from build123d import *


with BuildPart() as f1:
    # F0 (on Front) → F1 (revolve)
    with BuildSketch(Plane.XZ):
        with BuildLine():
            ThreePointArc((-1.815014, 4.25), (-1.448898, 3.366117), (-0.565014, 3))
            Line((-0.565014, 3), (6.184986, 3))
            Line((6.184986, 3), (6.184986, 3.909007))
            Line((6.184986, 3.909007), (5.934986, 4))
            Line((5.934986, 4), (-0.565014, 4))
            ThreePointArc((-0.565014, 4), (-0.741791, 4.073223), (-0.815014, 4.25))
            Line((-0.815014, 4.25), (-0.815014, 6))
            Line((-0.815014, 6), (-1.815014, 6))
            Line((-1.815014, 6), (-1.815014, 4.25))
        make_face()
    revolve(axis=Axis((-0.667828, 0, 0), (1, 0, 0)))


solid = f1.part
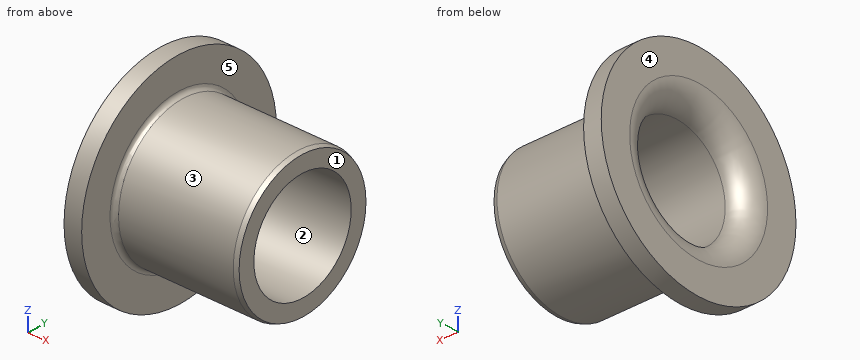
CAD build for the part. Positions are in the model's coordinates, mm. Face numbers are marked on the shaded views. A direction names the side the tool comes from. Give positions to 0.01 mm unless a question says otherwise; leave off trailing zeros. Order: outer loops, then holes, each group sorted by start corner. A loop starts at its lowest first (then second) coordinate and runs counter-clockwise, first axis right, second up. Notation, with made-up numbers: (-31.75, -0.75) - (2.25, -0.75) arc R28 ccw to (2.25, 19.25) - close; hole circle Ø4 at (82, 36.25). An arc over 180 degrees is marked (long way). Answer in a Markdown table with one row per item.
1. Saw through at A-A, the plane y = 0. Give the cut face in (x, z).
Data:
| item | result |
|---|---|
| outline | (-1.82, -6) - (-0.82, -6) - (-0.82, -4.25) arc R0.25 cw to (-0.57, -4) - (5.93, -4) - (6.18, -3.91) - (6.18, -3) - (-0.57, -3) arc R1.25 ccw to (-1.82, -4.25) - close; (-1.82, 4.25) arc R1.25 ccw to (-0.57, 3) - (6.18, 3) - (6.18, 3.91) - (5.93, 4) - (-0.57, 4) arc R0.25 cw to (-0.82, 4.25) - (-0.82, 6) - (-1.82, 6) - close |
2. Saw through at C-C, the plane x = 0.5. Give the cut face in (y, z), plus the area to 3 significant figures.
Data:
| item | result |
|---|---|
| outline | circle Ø8 at (0, 0); hole circle Ø6 at (0, 0) |
| area | 22.0 mm² |
3. Tool access for the marked faces 4 and 5: list every direction of +Z, -Z, +X, -X, +Y, -Y with a clear straight run to the whole face (end or side of a thin tool).
Data:
| item | result |
|---|---|
| face 4 | +Z, -Z, -X, +Y, -Y |
| face 5 | +X |
4. Probe probe 1 along Z at (x, y) = (1.5, 0); probe 2 along X at (y, z) = (-3, 4.5). List the from-to ranges inside material, lowest first. Write a range as [from, to].
Data:
| item | result |
|---|---|
| probe 1 | z = [-4, -3], [3, 4] |
| probe 2 | x = [-1.82, -0.82] |
5. Saw through at D-D, the plane x = -1. Give the cut face in (y, z).
Data:
| item | result |
|---|---|
| outline | circle Ø12 at (0, 0); hole circle Ø6.16 at (0, 0) |
6. Pull direction Z, two halves, no side cores. Call the marked faces 1, 2 and 3: pulls with the +Z half, pulls with the -Z half, needs draft (parallel to the pull), parting line crosses it, or undercut.
Data:
| item | result |
|---|---|
| face 1 | needs draft |
| face 2 | undercut |
| face 3 | parting line crosses it |
7. Flat gauge pins, fed straight in: pin 1 (1 mm diameter, centred on x = 1.5, z = 0.5, fed in from +Y); pin 2 (3.5 mm diameter, centred on y = -1, z = 0.5, fed in from +X); pin 3 (3 mm diameter, centred on x = 4.5, y = -3, fed in from +Z). Where does each tip first touch, or does it go through?
Data:
| item | result |
|---|---|
| pin 1 | stops at y = 4 |
| pin 2 | passes through |
| pin 3 | stops at z = 3.71 |
